For this review, use the dimensioned drawing (mm, ordinates from the lowest corner) and the shaded views. A direction names the side the tool comes from. Coordinates: 2 decimals unless noted, no trailing zeros. Order: outer loops, then holes, each group sorted by start corner. A loop starts at its lowest first (then second) coordinate and runs counter-clockwise, first axis right, second up. Notation, with made-up numbers: M 9.25,8 L 24.25,8 A16 ccw 24.25,12 Z; hole C -10,-34.5 d1. An arc over 180 degrees is marked long. Write each question's results on one line, items separated by ' | '.
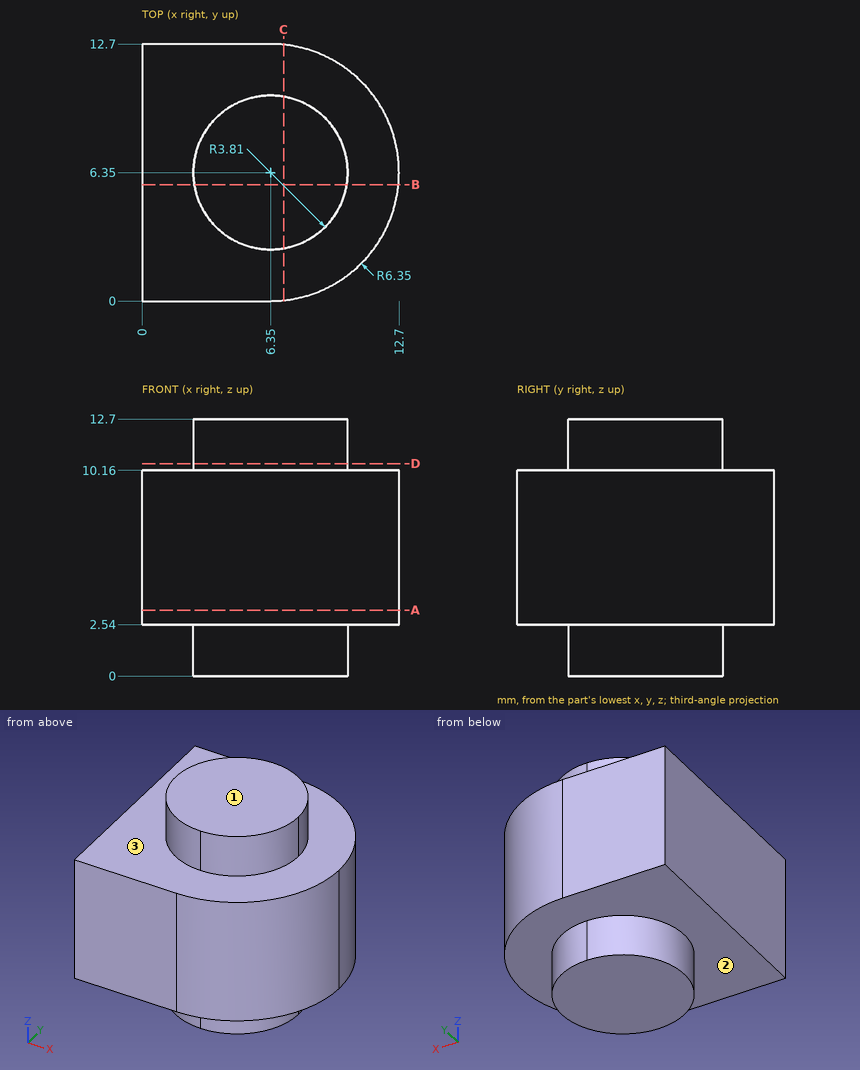
1) For the marked faces 1, 2 and 3, list the 3-axis set-ups (+Z, -Z, +X, -X, +Y, -Y) from which the entire face can be reached by the end or side of a thin tool; tool diameter is ignored.
Solutions:
face 1: +Z, +X, -X, +Y, -Y | face 2: -Z | face 3: +Z
2) Take a section at C-C on x = 7. State the section outline as (y, z) points, plus the area to 3 significant figures.
Solutions:
outline: M 0.03,2.54 L 2.6,2.54 L 2.6,0 L 10.1,0 L 10.1,2.54 L 12.67,2.54 L 12.67,10.16 L 10.1,10.16 L 10.1,12.7 L 2.6,12.7 L 2.6,10.16 L 0.03,10.16 Z | area: 134 mm2
3) Take a section at A-A on z = 3.25. State the section outline as (x, y) points.
Solutions:
outline: M 0,0 L 6.35,0 A6.35 ccw 6.35,12.7 L 0,12.7 Z
4) Take a section at B-B on y = 5.75. State the section outline as (x, z) points, plus the area to 3 significant figures.
Solutions:
outline: M 0,2.54 L 2.59,2.54 L 2.59,0 L 10.11,0 L 10.11,2.54 L 12.67,2.54 L 12.67,10.16 L 10.11,10.16 L 10.11,12.7 L 2.59,12.7 L 2.59,10.16 L 0,10.16 Z | area: 135 mm2
5) Take a section at D-D on z = 10.5. State the section outline as (x, y) points.
Solutions:
outline: C 6.35,6.35 d7.62
6) To check wall thickness, follow line 1 along Y through (x, z) = (6.5, 12); line 2 along X through (y, z) = (6.5, 9.25). State the ranges of each line that lie inside material, in increasing order.
Solutions:
line 1: 2.54 to 10.16 | line 2: 0 to 12.7
7) For pin 1 (5 mm diameter, centred on y = 11.5, z = 4.5, fed in from -X); pin 2 (1 mm diameter, centred on x = 11, z = 8.5, fed in from +Y), all flat-tipped, find the tip position at first contact; note any pin that passes through.
Solutions:
pin 1: x = 0 | pin 2: y = 11.16
